Geometry: see drawing. Coordinates: mm, zero at the bounding-box minimum. Round coordinates to 2 decimals unless told otherwise and drop trailing zeros. Loops run counter-clockwise (first coordinate to the right, second up) from the corner with the lowest first, then second, coordinate; pieces in that order, holes last. Notation, with made-up numbers: (33, 70.5) - (74, 70.5) arc R13 ccw to (74, 88.5) - close; hole circle Ø6 at (24.25, 77.5). An arc over 180 degrees is marked (long way). Return JSON: item names as keys, results as strings. Group by question number.
1. Material intervals for probe 1 along Y at (x, z) = (250, 11.5); probe 2 along Y at (x, z) = (597.5, 4); probe 3 along Y at (x, z) = (120, 7.5), sorted ascending.
2. Section C-C on z = 9.5. Return loops of the section in (x, y).
3. Section B-B on x = 597.5. Return loops of the section in (y, z), and give its area (4 significant figures).
4. Section D-D on y = 581. Return loops of the section in (x, z).
5. Section A-A on y = 397.5. Return loops of the section in (x, z), and give its area (3 significant figures).
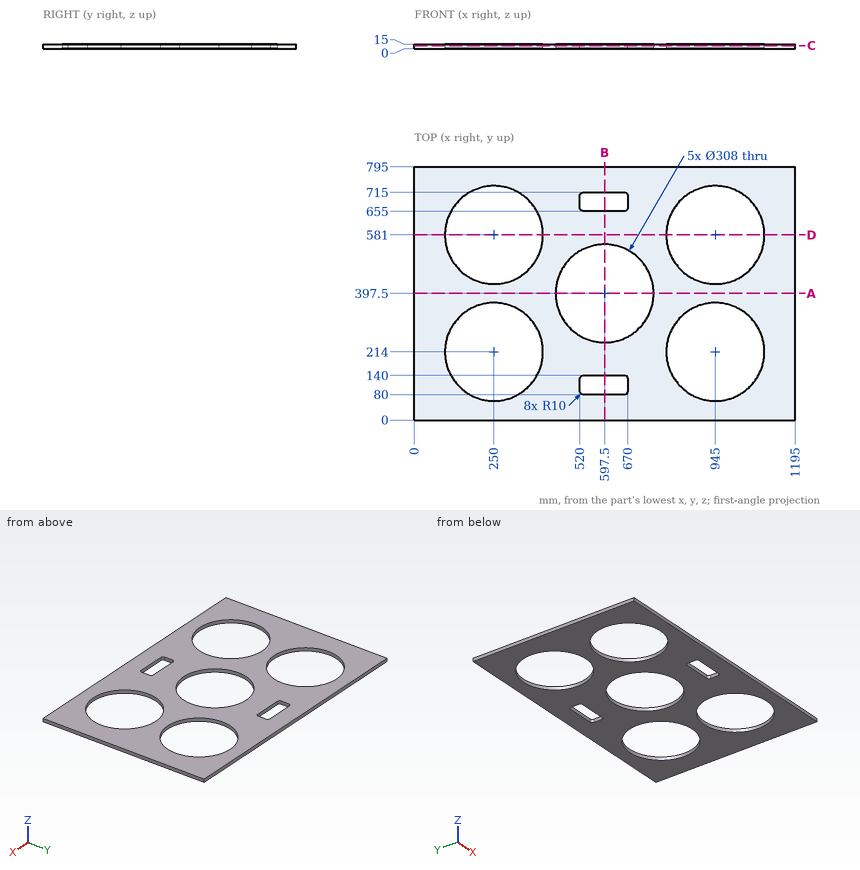
Taken from the geometry:
{
 "1": {"probe 1": "0 to 60, 368 to 427, 735 to 795", "probe 2": "0 to 80, 140 to 243.5, 551.5 to 655, 715 to 795", "probe 3": "0 to 131.44, 296.56 to 498.44, 663.56 to 795"},
 "2": {"outline": "(0, 0) - (1195, 0) - (1195, 795) - (0, 795) - close; hole circle Ø308 at (250, 214); hole circle Ø308 at (250, 581); hole circle Ø308 at (597.5, 397.5); hole (520, 90) arc R10 ccw to (530, 80) - (660, 80) arc R10 ccw to (670, 90) - (670, 130) arc R10 ccw to (660, 140) - (530, 140) arc R10 ccw to (520, 130) - close; hole (520, 665) arc R10 ccw to (530, 655) - (660, 655) arc R10 ccw to (670, 665) - (670, 705) arc R10 ccw to (660, 715) - (530, 715) arc R10 ccw to (520, 705) - close; hole circle Ø308 at (945, 214); hole circle Ø308 at (945, 581)"},
 "3": {"outline": "(0, 0) - (80, 0) - (80, 15) - (0, 15) - close; (140, 0) - (243.5, 0) - (243.5, 15) - (140, 15) - close; (551.5, 0) - (655, 0) - (655, 15) - (551.5, 15) - close; (715, 0) - (795, 0) - (795, 15) - (715, 15) - close", "area": "5,505 mm2"},
 "4": {"outline": "(0, 0) - (96, 0) - (96, 15) - (0, 15) - close; (404, 0) - (791, 0) - (791, 15) - (404, 15) - close; (1099, 0) - (1195, 0) - (1195, 15) - (1099, 15) - close"},
 "5": {"outline": "(0, 0) - (443.5, 0) - (443.5, 15) - (0, 15) - close; (751.5, 0) - (1195, 0) - (1195, 15) - (751.5, 15) - close", "area": "13,300 mm2"}
}
